```python
from build123d import *

# Parameters (mm, degrees)
EXTRUDE_1_DEPTH             = 50
SKETCH_2_W                  = 36
SKETCH_2_H                  = 102.163867091
CUT_EXTRUDE_1_DEPTH         = 43
HOLE_WIZARD_1_8_1_8_1_D     = 1.8
HOLE_WIZARD_1_8_1_8_1_DEPTH = 7
HOLE_WIZARD_M30_1_D         = 32
HOLE_WIZARD_M30_1_DEPTH     = 7
HOLE_WIZARD_M30_2_D         = 32
HOLE_WIZARD_M30_2_DEPTH     = 7
SKETCH_13_R                 = 1.4
CUT_EXTRUDE_2_DEPTH         = 10
SKETCH_14_R                 = 1.4
CUT_EXTRUDE_3_DEPTH         = 4


with BuildPart() as part:
    # 스케치1 → 보스-돌출1 (new body)
    with BuildSketch(Plane(origin=(-75, 0, 0), x_dir=(0, -1, 0), z_dir=(-1, 0, 0))):
        with BuildLine():
            Line((-21, 0), (-21, -45))
            Line((-21, -45), (21, -45))
            Line((21, -45), (21, 0))
            ThreePointArc((21, 0), (0, 21), (-21, 0))
        make_face()
    extrude(amount=-EXTRUDE_1_DEPTH)

    # 스케치2 → 컷-돌출1 (cut, through all)
    with BuildSketch(Plane(origin=(0, 21, 0), x_dir=(-1, 0, 0), z_dir=(0, 1, 0))):
        with Locations((50, 13.081933546)):
            Rectangle(SKETCH_2_W, SKETCH_2_H)
    extrude(amount=-CUT_EXTRUDE_1_DEPTH, mode=Mode.SUBTRACT)

    # Ø1.8 (1.8) 지름 구멍1
    with Locations(Plane(origin=(0, 0, -45), x_dir=(-1, 0, 0), z_dir=(0, 0, -1))):
        with Locations((35.3332236, 10), (65.3332236, 10), (35.3332236, -10), (65.3332236, -10)):
            Hole(HOLE_WIZARD_1_8_1_8_1_D / 2, depth=HOLE_WIZARD_1_8_1_8_1_DEPTH)

    # M30 여유 구멍1
    with Locations(Plane(origin=(-25, 0, 0), x_dir=(0, 0, -1), z_dir=(1, 0, 0))):
        with Locations((0, 0)):
            Hole(HOLE_WIZARD_M30_1_D / 2, depth=HOLE_WIZARD_M30_1_DEPTH)

    # M30 여유 구멍2
    with Locations(Plane.ZY.offset(75)):
        with Locations((0, 0)):
            Hole(HOLE_WIZARD_M30_2_D / 2, depth=HOLE_WIZARD_M30_2_DEPTH)

    # 스케치13 → 컷-돌출2 (cut)
    with BuildSketch(Plane.XY.offset(-38)):
        with Locations((-50.876817985, -16)):
            Circle(SKETCH_13_R)
        with Locations((-50.876817985, 16)):
            Circle(SKETCH_13_R)
    extrude(amount=-CUT_EXTRUDE_2_DEPTH, mode=Mode.SUBTRACT)

    # 스케치14 → 컷-돌출3 (cut)
    with BuildSketch(Plane(origin=(-25, 0, 0), x_dir=(0, 0, -1), z_dir=(1, 0, 0))):
        with Locations((41.267143481, 16.25)):
            Circle(SKETCH_14_R)
        with Locations((41.267143481, -16.25)):
            Circle(SKETCH_14_R)
    cut_extrude_3 = extrude(amount=-CUT_EXTRUDE_3_DEPTH, mode=Mode.SUBTRACT)

    # 대칭 복사1: 컷-돌출3 across plane
    add(cut_extrude_3.mirror(Plane.ZY.offset(50)), mode=Mode.SUBTRACT)


solid = part.part
```
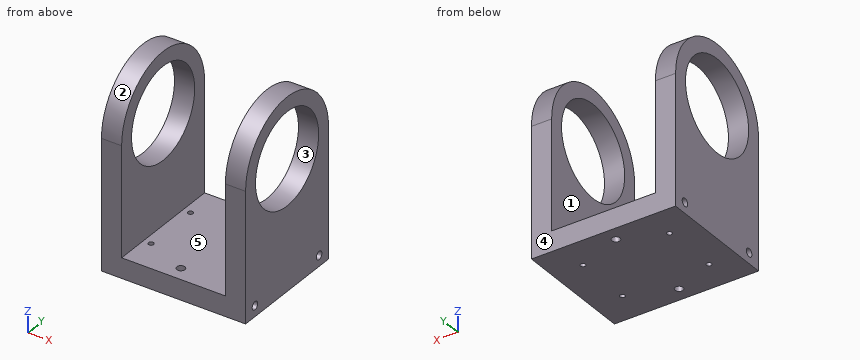
The model under review builds one solid part; all positions refer to its coordinate system, in mm. Face numbers are marked on the shaded views. A direction names the side the tool comes from. Round coordinates to 2 decimals unless told otherwise and drop trailing zeros. Order: outer loops, then holes, each group sorted by start corner. A loop starts at its lowest first (then second) coordinate and runs counter-clockwise, first axis right, second up. Notation, with made-up numbers: (73.5, -31) -> (127.5, -31) arc R27 cw to (127.5, -9) -> close; hole circle Ø2 at (24.5, -11). An arc over 180 degrees is marked (long way). One line per item, written item: value. Start each with the question number.
Q1. Machinability: for the marked faces 1 and 2, which of the approach directions +Z, -Z, +X, -X, +Y, -Y give a long, thin tool a straight path to every point of the face, cutting with its end or side? Answer none if there is none.
Q2. Wall thickness on line 1 (X direction, y = -6, z = -25); line 2 (Y direction, x = -72, z = 0); line 3 (Z direction, x = -49, y = 7): over which ranges is each line inside the solid? List them lowest first.
Q3. Clearance check with flat-ended pins moving along their axes: pin 1 Ø1.7 at (y, z) = (16.25, -41.27) entering from -X; pin 2 Ø8 at (x, z) = (-63.5, 9.5) entering from -Y; pin 3 Ø6 at (x, y) = (-58.5, 14) entering from +Z; pin 4 Ø2 at (y, z) = (-16.5, -41) entering from +X. State where each tip first meets the part, or that it passes through.
Q4. Take a section at B-B (z = 14.5). Write out the cut boundary in (x, y), and give its area (3 significant figures).
Q5. Take a section at D-D (z = -36). Write out the cut boundary in (x, y).
Q6. Mouldability with a two-part tool opening along Y and no side actions: class the marked faces 3, 4 and 5 as released by +Y, released by -Y, zero draft, split by the parting line, or undercut.
Q7. Take a section at C-C (x = -31). Write out the cut boundary in (y, z), and give its area (3 significant figures).
Q8. Take a section at A-A (y = 0). Write out the cut boundary in (x, z).
Reported:
1. face 1: +Z, +Y, -Y
1. face 2: +Z, +X, -X
2. line 1: x = -75 to -68, -32 to -25
2. line 2: y = -21 to -16, 16 to 21
2. line 3: z = -45 to -38
3. pin 1: stops at x = -71
3. pin 2: passes through
3. pin 3: stops at z = -38
3. pin 4: stops at x = -29
4. outline: (-75, -15.19) -> (-68, -15.19) -> (-68, -6.76) -> (-75, -6.76) -> close; (-75, 6.76) -> (-68, 6.76) -> (-68, 15.19) -> (-75, 15.19) -> close; (-32, -15.19) -> (-25, -15.19) -> (-25, -6.76) -> (-32, -6.76) -> close; (-32, 6.76) -> (-25, 6.76) -> (-25, 15.19) -> (-32, 15.19) -> close
4. area: 236 mm2
5. outline: (-75, -21) -> (-68, -21) -> (-68, 21) -> (-75, 21) -> close; (-32, -21) -> (-25, -21) -> (-25, 21) -> (-32, 21) -> close
6. face 3: undercut
6. face 4: released by +Y
6. face 5: zero draft
7. outline: (-21, -45) -> (21, -45) -> (21, 0) arc R21 ccw to (-21, 0) -> close; hole circle Ø32 at (0, 0)
7. area: 1,780 mm2
8. outline: (-75, -45) -> (-25, -45) -> (-25, -16) -> (-32, -16) -> (-32, -38) -> (-68, -38) -> (-68, -16) -> (-75, -16) -> close; (-75, 16) -> (-68, 16) -> (-68, 21) -> (-75, 21) -> close; (-32, 16) -> (-25, 16) -> (-25, 21) -> (-32, 21) -> close
